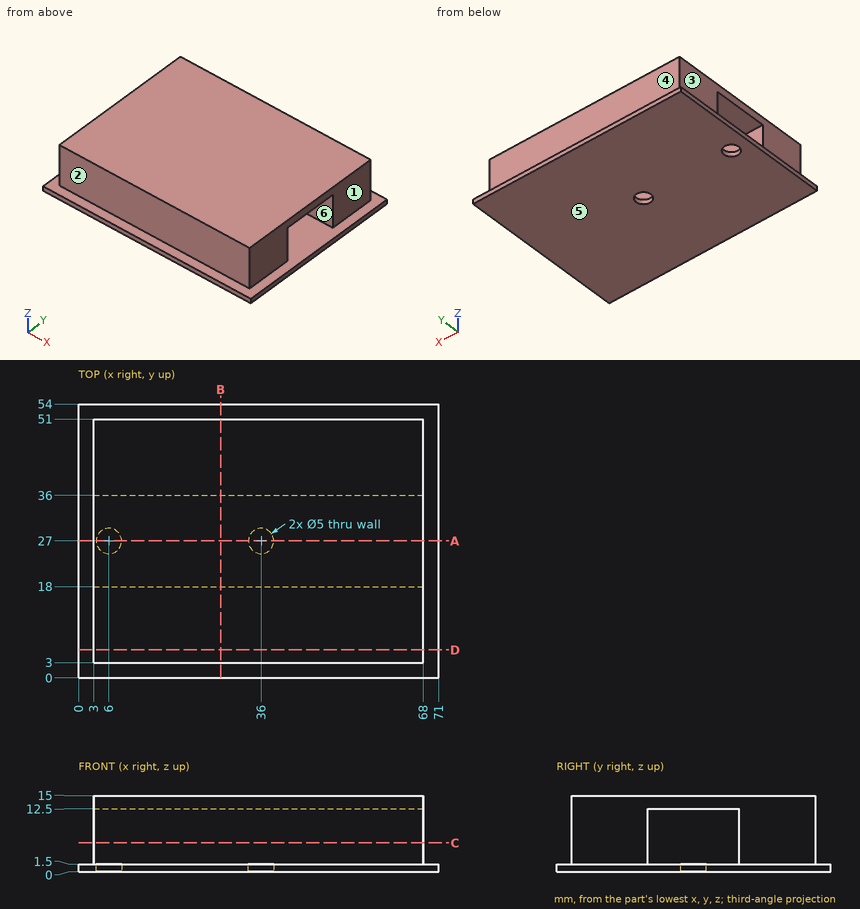
Study the drawing (mm; zero at the part's minimum x, y, z) and answer. A direction names the side the tool comes from. Round coordinates to 2 decimals unless told otherwise and drop trailing zeros. Order: outer loops, then holes, each group sorted by start corner. A loop starts at its lowest first (then second) coordinate and runs counter-clockwise, first axis right, second up. Notation, with made-up numbers: (-13.75, 79) -> (22.25, 79) arc R23 ccw to (22.25, 93) -> close; hole circle Ø1 at (-36.75, -9). An arc over 180 degrees is marked (long way). Write each question's results on one line, items separated by ' | '. Start each with the question number.
Q1. Straight lines are drawn through the part: probe 1 along Y at (x, z) = (36, 0.3); probe 2 along Y at (x, z) = (14, 10.5); probe 3 along Z at (x, y) = (39.5, 31). For each, find the intervals that lie inside material, in ascending order. Write a range as from..to.
Q2. Find section D-D (y = 5.5). Determine the outline of the cut face in (x, z), then the cut area to 3 significant figures.
Q3. Find section A-A (y = 27). Determine the outline of the cut face in (x, z), then the cut area to 3 significant figures.
Q4. Each of these flat-tipped pins is pushed along its axis until it touches: pin 1 (8 mm diameter, centred on y = 5.5, z = 8.5, fed in from +X); pin 2 (6 mm diameter, centred on x = 36, y = 27, fed in from -Z); pin 3 (9 mm diameter, centred on x = 45.5, z = 6.5, fed in from -Y). Where does it stop, or does it pass through?
Q5. Find section C-C (z = 5.75). Determine the outline of the cut face in (x, y).
Q6. The mould has two halves that part along Z. Classify the marked faces 4, 5 and 6: pulls with the +Z half, pulls with the -Z half, needs draft (parallel to the pull), parting line crosses it, or undercut.
Q7. Which of the six approach directions +Z, -Z, +X, -X, +Y, -Y give full straight-line access (tool end or side, diameter ignored) to the marked faces 1, 2 and 3?
Q8. Find section B-B (x = 28). Determine the outline of the cut face in (y, z), then the cut area to 3 significant figures.
Worked answers:
1) probe 1: y = 0..24.5, 29.5..54 | probe 2: y = 3..18, 36..51 | probe 3: z = 0..1.5, 12.5..15
2) outline: (0, 0) -> (71, 0) -> (71, 1.5) -> (68, 1.5) -> (68, 15) -> (3, 15) -> (3, 1.5) -> (0, 1.5) -> close | area: 984 mm2
3) outline: (0, 0) -> (3.5, 0) -> (3.5, 1.5) -> (0, 1.5) -> close; (3, 12.5) -> (68, 12.5) -> (68, 15) -> (3, 15) -> close; (8.5, 0) -> (33.5, 0) -> (33.5, 1.5) -> (8.5, 1.5) -> close; (38.5, 0) -> (71, 0) -> (71, 1.5) -> (38.5, 1.5) -> close | area: 254 mm2
4) pin 1: stops at x = 68 | pin 2: stops at z = 0 | pin 3: stops at y = 3
5) outline: (3, 3) -> (68, 3) -> (68, 18) -> (3, 18) -> close; (3, 36) -> (68, 36) -> (68, 51) -> (3, 51) -> close
6) face 4: needs draft | face 5: pulls with the -Z half | face 6: undercut
7) face 1: +Z, +X, +Y, -Y | face 2: +Z, +X, -X, -Y | face 3: +Z, -X, +Y, -Y
8) outline: (0, 0) -> (54, 0) -> (54, 1.5) -> (51, 1.5) -> (51, 15) -> (3, 15) -> (3, 1.5) -> (0, 1.5) -> close; hole (18, 1.5) -> (36, 1.5) -> (36, 12.5) -> (18, 12.5) -> close | area: 531 mm2
